Job drawing, mm, ordinate dimensions from the low corner. One solid piece. A direction names the side the tool comes from. Coordinates: 2 decimals unless noted, no trailing zeros. Order: outer loops, then holes, each group sorted by start corner. A loop starts at its lowest first (then second) coordinate and runs counter-clockwise, first axis right, second up. Notation, with made-up numbers: M -25,10.5 L 1,10.5 A19 ccw 1,30.5 Z; hole C -22,11 d11. An arc over 180 degrees is marked long. Write item = value, one per line.
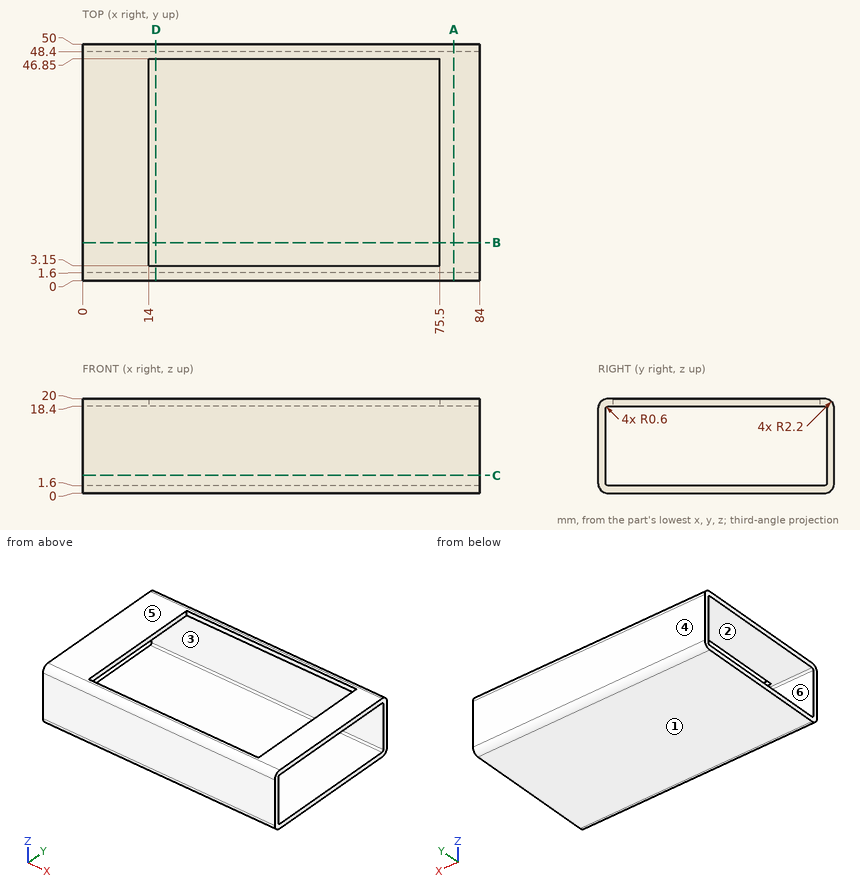
(1) Pull direction Z, two halves, no side cores. Call the marked faces 3, 4, 5 and 6: +Z half, -Z half, draft (parallel to the pull), parting line (faces both ways), or undercut.
Evaluation:
face_3 = undercut
face_4 = draft
face_5 = +Z half
face_6 = undercut
(2) Wall check: line 1 (Y direction, x = 9, z = 2.75); line 2 (Z direction, x = 80, y = 4.5); line 3 (Z direction, x = 32.5, y = 39.5). Give the ranges that are in metal, low to high. Write a range as from..to.
Evaluation:
line_1 = 0..1.6, 48.4..50
line_2 = 0..1.6, 18.4..20
line_3 = 0..1.6
(3) Slice it at D-D, the plane x = 15.5. Write the cut outline in (y, z).
Evaluation:
outline = M 0,2.2 A2.2 ccw 2.2,0 L 47.8,0 A2.2 ccw 50,2.2 L 50,17.8 A2.2 ccw 47.8,20 L 46.85,20 L 46.85,18.4 L 47.8,18.4 A0.6 cw 48.4,17.8 L 48.4,2.2 A0.6 cw 47.8,1.6 L 2.2,1.6 A0.6 cw 1.6,2.2 L 1.6,17.8 A0.6 cw 2.2,18.4 L 3.15,18.4 L 3.15,20 L 2.2,20 A2.2 ccw 0,17.8 Z
(4) Slice it at C-C, the plane z = 3.75. Write the cut outline in (x, y).
Evaluation:
outline = M 0,0 L 84,0 L 84,1.6 L 0,1.6 Z; M 0,48.4 L 84,48.4 L 84,50 L 0,50 Z
(5) Tool access for the marked faces 1 and 2: list every direction of +Z, -Z, +X, -X, +Y, -Y with a clear straight run to the whole face (end or side of a thin tool).
Evaluation:
face_1 = -Z, +X, -X, +Y, -Y
face_2 = +X, -X
(6) Slice it at B-B, the plane y = 8. Write the cut outline in (x, z).
Evaluation:
outline = M 0,0 L 84,0 L 84,1.6 L 0,1.6 Z; M 0,18.4 L 14,18.4 L 14,20 L 0,20 Z; M 75.5,18.4 L 84,18.4 L 84,20 L 75.5,20 Z
(7) Slice it at A-A, the plane x = 78.5. Write the cut outline in (y, z), then the cut area to 3 significant figures.
Evaluation:
outline = M 0,2.2 A2.2 ccw 2.2,0 L 47.8,0 A2.2 ccw 50,2.2 L 50,17.8 A2.2 ccw 47.8,20 L 2.2,20 A2.2 ccw 0,17.8 Z; hole M 1.6,2.2 A0.6 ccw 2.2,1.6 L 47.8,1.6 A0.6 ccw 48.4,2.2 L 48.4,17.8 A0.6 ccw 47.8,18.4 L 2.2,18.4 A0.6 ccw 1.6,17.8 Z
area = 210 mm²
(8) Pin check, flat tips, straight feed: pin 1 Ø1.8 at (y, z) = (33.5, 19.5) entering from -X; pin 2 Ø1.5 at (y, z) = (5.5, 16) entering from -X; pin 3 Ø1.8 at (x, z) = (45, 19) entering from -Y; pin 4 Ø5 at (x, y) = (44, 7.5) entering from +Z. Stop position of each tip, or through.
Evaluation:
pin_1 = 0
pin_2 = through
pin_3 = 0.02
pin_4 = 1.6
